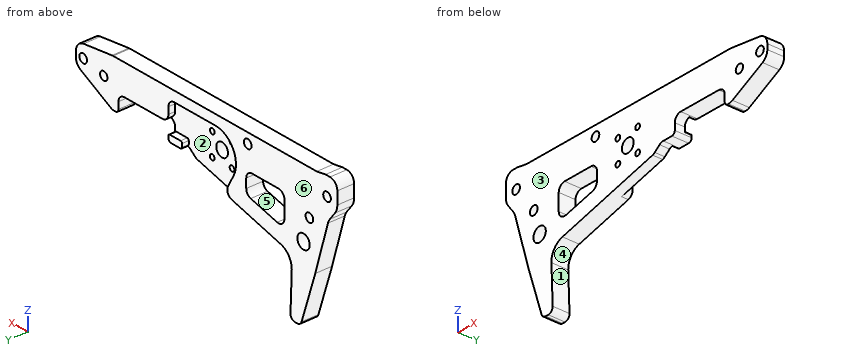
```python
from build123d import *

# Parameters (mm, degrees)
SKETCH1_R           = 2.6
SKETCH1_R_2         = 4.2
SKETCH1_R_3         = 2.5
BOSS_EXTRUDE1_DEPTH = 10
FILLET2_R           = 6
FILLET3_R           = 3
CUT_EXTRUDE1_DEPTH  = 11
SKETCH7_R           = 2.6
CUT_EXTRUDE4_DEPTH  = 11
FILLET8_R           = 5
FILLET9_R           = 4
SKETCH10_W          = 34
SKETCH10_H          = 10
CUT_EXTRUDE6_DEPTH  = 11
FILLET11_R          = 2
CUT_EXTRUDE7_DEPTH  = 4
FILLET13_R          = 10
FILLET14_R          = 4
FILLET15_R          = 1
FILLET16_R          = 4
FILLET17_R          = 4
SKETCH13_R          = 4
CUT_EXTRUDE8_DEPTH  = 10
FILLET19_R          = 8
SKETCH14_R          = 1.6
CUT_EXTRUDE9_DEPTH  = 10


with BuildPart() as part:
    # Sketch1 → Boss-Extrude1 (new body)
    with BuildSketch(Plane(origin=(0, 0, 0), x_dir=(1, 0, 0), z_dir=(0, 1, 0))):
        Polygon((164, 15), (139, 28), (91.716233646, 28), (86.716233646, 32), (16.716233646, 50), (18, 84), (11, 84), (1, 53), (-8, 22), (-14, 14), (-14, 2), (-14, -1), (-6, -1), (0, 0), (139, 0), (164, 3), align=None)
        with Locations((-7, 10)):
            Circle(SKETCH1_R, mode=Mode.SUBTRACT)
        with Locations((159, 10)):
            Circle(SKETCH1_R, mode=Mode.SUBTRACT)
        with Locations((5, 26)):
            Circle(SKETCH1_R, mode=Mode.SUBTRACT)
        with Locations((9, 40)):
            Circle(SKETCH1_R_2, mode=Mode.SUBTRACT)
        with Locations((145, 13)):
            Circle(SKETCH1_R_3, mode=Mode.SUBTRACT)
    extrude(amount=BOSS_EXTRUDE1_DEPTH)

    # Fillet2
    fillet2_edges = [part.edges().sort_by_distance(p)[0] for p in [
        (139, 5, -28),
        (164, 5, -15),
        (164, 5, -3),
        (139, 5, 0),
    ]]
    fillet(fillet2_edges, radius=FILLET2_R)

    # Fillet3
    fillet3_edges = [part.edges().sort_by_distance(p)[0] for p in [
        (11, 5, -84),
        (18, 5, -84),
    ]]
    fillet(fillet3_edges, radius=FILLET3_R)

    # Sketch4 → Cut-Extrude1 (cut, through all)
    with BuildSketch(Plane(origin=(0, 10, 0), x_dir=(1, 0, 0), z_dir=(0, 1, 0))):
        Polygon((22, 39), (22, 20), (48, 20), (48, 32.5), align=None)
    extrude(amount=-CUT_EXTRUDE1_DEPTH, mode=Mode.SUBTRACT)

    # Sketch7 → Cut-Extrude4 (cut, through all)
    with BuildSketch(Plane(origin=(0, 10, 0), x_dir=(1, 0, 0), z_dir=(0, 1, 0))):
        with Locations((47, 6)):
            Circle(SKETCH7_R)
    extrude(amount=-CUT_EXTRUDE4_DEPTH, mode=Mode.SUBTRACT)

    # Fillet8
    fillet8_edges = [part.edges().sort_by_distance(p)[0] for p in [
        (-14, 5, 1),
    ]]
    fillet(fillet8_edges, radius=FILLET8_R)

    # Fillet9
    fillet9_edges = [part.edges().sort_by_distance(p)[0] for p in [
        (22, 5, -39),
        (48, 5, -32.5),
        (48, 5, -20),
        (22, 5, -20),
    ]]
    fillet(fillet9_edges, radius=FILLET9_R)

    # Sketch10 → Cut-Extrude6 (cut, through all)
    with BuildSketch(Plane(origin=(0, 10, 0), x_dir=(1, 0, 0), z_dir=(0, 1, 0))):
        with Locations((118, 23)):
            Rectangle(SKETCH10_W, SKETCH10_H)
    extrude(amount=-CUT_EXTRUDE6_DEPTH, mode=Mode.SUBTRACT)

    # Fillet11
    fillet11_edges = [part.edges().sort_by_distance(p)[0] for p in [
        (101, 5, -28),
        (135, 5, -28),
    ]]
    fillet(fillet11_edges, radius=FILLET11_R)

    # Sketch12 → Cut-Extrude7 (cut)
    with BuildSketch(Plane(origin=(0, 10, 0), x_dir=(1, 0, 0), z_dir=(0, 1, 0))):
        with BuildLine():
            Line((86.716233646, 32), (91.716233646, 28))
            Line((91.716233646, 28), (91.716233646, 24))
            Line((91.716233646, 24), (101, 24))
            Line((101, 24), (101, 6))
            Line((101, 6), (69, 6))
            ThreePointArc((69, 6), (57.064930536, 12.681932162), (56.522621715, 26.349411873))
            Line((56.522621715, 26.349411873), (62.882866971, 38.128580002))
            Line((62.882866971, 38.128580002), (86.716233646, 32))
        make_face()
    extrude(amount=-CUT_EXTRUDE7_DEPTH, mode=Mode.SUBTRACT)

    # Fillet13
    fillet13_edges = [part.edges().sort_by_distance(p)[0] for p in [
        (16.716233646, 5, -50),
    ]]
    fillet(fillet13_edges, radius=FILLET13_R)

    # Fillet14
    fillet14_edges = [part.edges().sort_by_distance(p)[0] for p in [
        (86.716233646, 3, -32),
        (91.716233646, 3, -28),
    ]]
    fillet(fillet14_edges, radius=FILLET14_R)

    # Fillet15
    fillet15_edges = [part.edges().sort_by_distance(p)[0] for p in [
        (91.716233646, 8, -24),
        (101, 8, -24),
        (91.716233646, 8, -28),
    ]]
    fillet(fillet15_edges, radius=FILLET15_R)

    # Fillet16
    fillet16_edges = [part.edges().sort_by_distance(p)[0] for p in [
        (101, 8, -18),
        (62.882866971, 8, -38.128580002),
    ]]
    fillet(fillet16_edges, radius=FILLET16_R)

    # Fillet17
    fillet17_edges = [part.edges().sort_by_distance(p)[0] for p in [
        (101, 3, -18),
        (101, 8, -6),
        (135, 5, -18),
    ]]
    fillet(fillet17_edges, radius=FILLET17_R)

    # Sketch13 → Cut-Extrude8 (cut)
    with BuildSketch(Plane(origin=(0, 6, 0), x_dir=(1, 0, 0), z_dir=(0, 1, 0))):
        with Locations((69, 20)):
            Circle(SKETCH13_R)
    extrude(amount=-CUT_EXTRUDE8_DEPTH, mode=Mode.SUBTRACT)

    # Fillet19
    fillet19_edges = [part.edges().sort_by_distance(p)[0] for p in [
        (-14, 5, -14),
        (-8, 5, -22),
    ]]
    fillet(fillet19_edges, radius=FILLET19_R)

    # Sketch14 → Cut-Extrude9 (cut)
    with BuildSketch(Plane(origin=(0, 6, 0), x_dir=(1, 0, 0), z_dir=(0, 1, 0))):
        with Locations((62.3, 26.734983296)):
            Circle(SKETCH14_R)
        with Locations((75.734983296, 26.7)):
            Circle(SKETCH14_R)
        with Locations((75.7, 13.265016704)):
            Circle(SKETCH14_R)
        with Locations((62.265016704, 13.3)):
            Circle(SKETCH14_R)
    extrude(amount=-CUT_EXTRUDE9_DEPTH, mode=Mode.SUBTRACT)


solid = part.part
```
Model file for the job. Use its own axes, mm. Face numbers are marked on the shaded views. A direction names the side the tool comes from. Give positions to 0.01 mm unless a question says otherwise; leave off trailing zeros. Write each loop counter-clockwise with the first axis right and the second up, starting at its lowest first coordinate (ties: lowest second). Pieces come first, ordered by that corner, then holes. Notation, with made-up numbers: (-2, -23) -> (24, -23) arc R30 cw to (24, 0) -> close; hole circle Ø7 at (60, 20). An arc over 180 degrees is marked (long way). Use CSV: the item, a comma, the result in double quotes. Start each with the question number.
1) Two-plate mould, pull along X, no slides. Class the marked faces 1, 2 and 3: released by +X, released by -X, zero draft, split by the parting line, or undercut.
2) Cut at B-B on x = 115.5. List the corners of the cut face in (y, z), plus the area to 3 significant figures.
3) Cut at A-A on x = 145. List the corners of the cut face in (y, z).
4) Tool access for the marked faces 4, 5 and 6: list every direction of +Z, -Z, +X, -X, +Y, -Y with a clear straight run to the whole face (end or side of a thin tool).
5) Cut at D-D on y = 2. Count the separate pieces of the cut face and the enclosed holes in it, plus the area to 3 significant figures.
6) Pin check, flat tips, straight feed: P1, Ø6.5, axis at x = 9, z = -40, coming from the +Y side; P2, Ø6, axis at x = 72, z = -33.5, coming from the +Y side; P3, Ø1, axis at x = 86, z = -25.5, coming from the -Y side; P4, Ø4, axis at y = 8.5, z = -21.5, coming from the +X side. Stop position of each tip, or through.
7) Cut at C-C on z = -60. List the corners of the cut face in (x, y), plus the area to 3 significant figures.
8) Drill centre lines: L1, parallel to X at y = 7, z = -21; L2, parallel to X at y = 9.5, z = -13.5; L3, parallel to X at y = 3.75, z = -27. Where is each one in solid material? Low to high.
Final values:
1,face 1,"released by +X"
1,face 2,"undercut"
1,face 3,"zero draft"
2,outline,"(0, -18) -> (10, -18) -> (10, 0) -> (0, 0) -> close"
2,area,"180 mm2"
3,outline,"(0, -24.88) -> (10, -24.88) -> (10, -15.5) -> (0, -15.5) -> close; (0, -10.5) -> (10, -10.5) -> (10, -0.72) -> (0, -0.72) -> close"
4,face 4,"+X, +Y, -Y"
4,face 5,"+Y, -Y"
4,face 6,"+Z, -Z, +X, -X, +Y"
5,separate pieces,"1"
5,enclosed holes,"12"
5,area,"5,510 mm2"
6,P1,"passes through"
6,P2,"stops at y = 6"
6,P3,"stops at y = 0"
6,P4,"stops at x = 155.35"
7,outline,"(3.26, 0) -> (17.09, 0) -> (17.09, 10) -> (3.26, 10) -> close"
7,area,"138 mm2"
8,L1,"x = -8.75 to 23.35, 46.65 to 55.04, 134.87 to 152.46"
8,L2,"x = -13.7 to 56.6, 101 to 142.55, 147.45 to 163.6"
8,L3,"x = -6.55 to 2.6, 7.4 to 22, 48 to 60.72, 63.88 to 74.16, 77.31 to 100.73, 135.27 to 140.92"
